The figure shows three views and two pictorial views of one solid part (mm, origin at its lowest corner). Answer the questions. A direction names the side the tool comes from. Coordinates: 2 decimals unless noted, no trailing zeros. Loops run counter-clockwise (first coordinate to the right, second up) from the corner with the lowest first, then second, coordinate; pieces in that order, holes last.
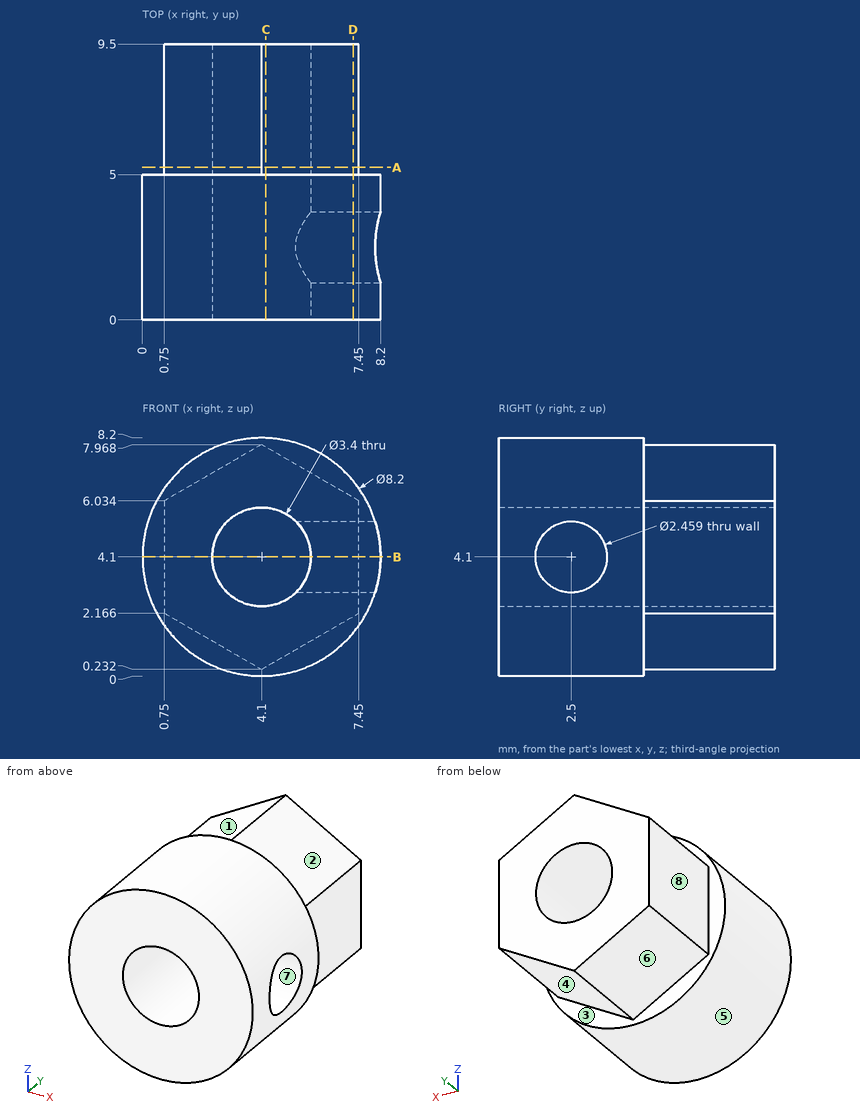
Q1. A cutting plane is placed at A-A (y = 5.25). Give the vertices of the cut face in (x, z).
Findings below:
outline: (0.75, 2.17) - (4.1, 0.23) - (7.45, 2.17) - (7.45, 6.03) - (4.1, 7.97) - (0.75, 6.03) - close; hole circle Ø3.4 at (4.1, 4.1)
Q2. A cutting plane is placed at D-D (x = 7.25). Give the vertices of the cut face in (y, z).
Findings below:
outline: (0, 1.48) - (5, 1.48) - (5, 2.05) - (9.5, 2.05) - (9.5, 6.15) - (5, 6.15) - (5, 6.72) - (0, 6.72) - close; hole circle Ø2.46 at (2.5, 4.1)
Q3. Which of the six approach directions +Z, -Z, +X, -X, +Y, -Y give full straight-line access (tool end or side, diameter ignored) to the marked faces 1, 2, 3 and 4?
Findings below:
face 1: +Z, -X, +Y
face 2: +Z, +X, +Y
face 3: +Y
face 4: -Z, +X, +Y
Q4. A cutting plane is placed at B-B (z = 4.1). Give the vertices of the cut face in (x, y).
Findings below:
outline: (0, 0) - (2.4, 0) - (2.4, 9.5) - (0.75, 9.5) - (0.75, 5) - (0, 5) - close; (5.8, 0) - (8.2, 0) - (8.2, 1.27) - (5.8, 1.27) - close; (5.8, 3.73) - (8.2, 3.73) - (8.2, 5) - (7.45, 5) - (7.45, 9.5) - (5.8, 9.5) - close
Q5. A cutting plane is placed at C-C (x = 4.25). Give the vertices of the cut face in (y, z).
Findings below:
outline: (0, 0) - (5, 0) - (5, 0.32) - (9.5, 0.32) - (9.5, 2.41) - (0, 2.41) - close; (0, 5.79) - (9.5, 5.79) - (9.5, 7.88) - (5, 7.88) - (5, 8.2) - (0, 8.2) - close
Q6. Straight lines are drawn through the part: probe 1 along Y at (x, z) = (6.45, 4.1); probe 2 along X at (y, z) = (4.75, 4.1); probe 3 along X at (y, z) = (6, 4.1). For each, find the intervals that lie inside material, in ascending order.
Findings below:
probe 1: y = 0 to 1.27, 3.73 to 9.5
probe 2: x = 0 to 2.4, 5.8 to 8.2
probe 3: x = 0.75 to 2.4, 5.8 to 7.45
Q7. Flat-ended cylindrical pins translate along their axes: pin 1 Ø4 at (y, z) = (3.5, 1.5) entering from +X; pin 2 Ø3 at (y, z) = (8, 4) entering from -X. Find the tip coordinate at first contact, or state that the pin passes through.
Findings below:
pin 1: stops at x = 8.16
pin 2: stops at x = 0.75
Q8. Determine the mould class of the marked faces 5, 6, 7 and 8 for opening direction Z: +Z half, -Z half, draft (parallel to the pull), parting line (faces both ways), or undercut.
Findings below:
face 5: parting line
face 6: -Z half
face 7: undercut
face 8: draft
